Part model, mm, in its own coordinate system. A direction names the side the tool comes from. Give positions to 0.01 mm unless a question says otherwise; leave off trailing zeros. Write each loop counter-clockwise with the first axis right and the second up, starting at its lowest first coordinate (ties: lowest second). Pieces come first, ordered by that corner, then holes. Notation, with made-up numbers: (88.25, 33.5) - (105.25, 33.5) arc R27 cw to (105.25, 59.5) - close; hole circle Ø2 at (-11, 34.5). An arc over 180 degrees is marked (long way). Answer in a Markdown table with one row per item. Add a question column.
1. Band-saw the part on A-A on y = 45. Write the cut outline in (x, z), plus the area to 3 significant figures.
2. Band-saw the part on B-B on y = -60.18. Write the cut outline in (x, z).
3. Which spindle directions (+Z, -Z, +X, -X, +Y, -Y) get a long thin tool onto all of the face, cutting with end or side? Do faces 1 (the flat face through (-16, 17, -11)), 2 (the cylindrical face through (-16.507, 73.676, -13.218)), 3 (the cylindrical face through (-10.5, 64.9, -0.5)), 4 (the flat face through (16.49, 3.77, -7.83)). Say none if no direction does.
4. Band-saw the part on C-C on x = 3.5. Write the cut outline in (y, z), plus the area to 3 significant figures.
5. Drop flat-ended pins along their axis: pin 1 Ø12 at (x, y) = (-11, -49.5) entering from +Z; pin 2 Ø1.1 at (y, z) = (-62, -0.5) entering from -X; pin 3 Ø0.8 at (x, y) = (-16.5, 18) entering from +Z; pin 4 Ø1 at (x, z) = (16, -2.5) entering from -Y. Give the stop position or say it passes through.
6. Probe line 1 along X through (y, z) = (-70.18, -0.8); line 2 along X through (y, z) = (60, -7.75); line 3 along Z through (x, y) = (-12, -53.5). List the from-to ranges inside material, lowest first.
7. Pull direction Z, two halves, no side cores. Call faces 5 (the flat face through (-16.51, 3.77, -7.83)), 6 (the cylindrical face through (10.5, 25.1, -0.5)), 7 (the flat face through (14, 1, -1)): released by +Z, released by -Z, zero draft, split by the parting line, or undercut.
8. Band-saw the part on D-D on z = -12.75. Write the cut outline in (x, y), plus the area to 3 significant figures.
```python
from build123d import *

# Parameters (mm, degrees)
SKETCH1_R                  = 6.5
BASE_FLANGE1_DEPTH         = 1
FILLET1_R                  = 5
SKETCHED_START             = 16.78876
SKETCHED_BEND1_OUTLINE_W   = 115.36
SKETCHED_BEND1_OUTLINE_H   = 1
SKETCHED_BEND1_DEPTH       = 13.21124
SKETCHED_START_2           = -30
SKETCHED_BEND1_2_OUTLINE_W = 115.36
SKETCHED_BEND1_2_OUTLINE_H = 1
SKETCHED_BEND1_2_DEPTH     = 13.18876
SKETCHED_START_3           = 16
SKETCHED_BEND1_3_DEPTH     = 0.0274
SKETCHED_START_4           = -16.01124
SKETCHED_BEND1_4_DEPTH     = 0.01124
SKETCHED_START_5           = -17
SKETCHED_BEND1_5_DEPTH     = 2
SKETCHED_START_6           = 15
SKETCHED_BEND1_6_DEPTH     = 2
SKETCHED_START_7           = -40.18
SKETCHED_BEND1_7_DEPTH     = 115.36
F_4_CLEARANCE_HOLE1_D      = 3.2639
FILLET2_R                  = 1
F_6_CLEARANCE_HOLE2_D      = 3.7973
CUT_EXTRUDE1_DEPTH         = 10


with BuildPart() as part:
    # Base-Flange1: sheet metal written as solids
    # Sketch1 → Base-Flange1 (new body)
    with BuildSketch(Plane.XY):
        Polygon((-30, 75.18), (30, 75.18), (30, -40.18), (15, -40.18), (15, -75.18), (-15, -75.18), (-15, -40.18), (-30, -40.18), align=None)
        with Locations((0, -60.18)):
            Circle(SKETCH1_R, mode=Mode.SUBTRACT)
        Polygon((-26, 60.18), (-19, 54.18), (-19, 36.18), (-26, 30.18), align=None, mode=Mode.SUBTRACT)
        Polygon((-26, 24.18), (-19, 30.18), (-19, 0.18), (-26, 6.18), align=None, mode=Mode.SUBTRACT)
        Polygon((-26, -29.82), (-26, 0.18), (-19, -5.82), (-19, -23.82), align=None, mode=Mode.SUBTRACT)
        Polygon((19, -23.82), (26, -29.82), (26, 0.18), (19, -5.82), align=None, mode=Mode.SUBTRACT)
        Polygon((19, 0.18), (26, 6.18), (26, 24.18), (19, 30.18), align=None, mode=Mode.SUBTRACT)
        Polygon((19, 36.18), (26, 30.18), (26, 60.18), (19, 54.18), align=None, mode=Mode.SUBTRACT)
    extrude(amount=-BASE_FLANGE1_DEPTH)

    # Fillet1
    fillet1_edges = [part.edges().sort_by_distance(p)[0] for p in [
        (-30, 75.18, -0.5),
        (30, 75.18, -0.5),
        (30, -40.18, -0.5),
        (15, -75.18, -0.5),
        (-15, -75.18, -0.5),
        (-30, -40.18, -0.5),
    ]]
    fillet(fillet1_edges, radius=FILLET1_R)

    # Sketched Bend1: read off the stored shape, not the designer's step
    # Sketched Bend1 outline → Sketched Bend1 (cut)
    with BuildSketch(Plane.YZ.offset(SKETCHED_START)):
        with Locations((17.5, -0.5)):
            Rectangle(SKETCHED_BEND1_OUTLINE_W, SKETCHED_BEND1_OUTLINE_H)
    extrude(amount=SKETCHED_BEND1_DEPTH, mode=Mode.SUBTRACT)

    # Sketched Bend1 2 outline → Sketched Bend1 2 (cut)
    with BuildSketch(Plane.YZ.offset(SKETCHED_START_2)):
        with Locations((17.5, -0.5)):
            Rectangle(SKETCHED_BEND1_2_OUTLINE_W, SKETCHED_BEND1_2_OUTLINE_H)
    extrude(amount=SKETCHED_BEND1_2_DEPTH, mode=Mode.SUBTRACT)

    # Sketched Bend1 3 outline → Sketched Bend1 3 (add)
    with BuildSketch(Plane.YZ.offset(SKETCHED_START_3)):
        with BuildLine():
            Line((75.18, -9.64380551), (75.18, -1))
            Line((75.18, -1), (-40.18, -1))
            Line((-40.18, -1), (-40.18, -9.64380551))
            ThreePointArc((-40.18, -9.64380551), (-38.715533906, -13.179339416), (-35.18, -14.64380551))
            Line((-35.18, -14.64380551), (70.18, -14.64380551))
            ThreePointArc((70.18, -14.64380551), (73.715533906, -13.179339416), (75.18, -9.64380551))
        make_face()
        Polygon((-23.82, -3.64380551), (-5.82, -3.64380551), (0.18, -10.64380551), (-29.82, -10.64380551), align=None, mode=Mode.SUBTRACT)
        Polygon((0.18, -3.64380551), (30.18, -3.64380551), (24.18, -10.64380551), (6.18, -10.64380551), align=None, mode=Mode.SUBTRACT)
        Polygon((36.18, -3.64380551), (54.18, -3.64380551), (60.18, -10.64380551), (30.18, -10.64380551), align=None, mode=Mode.SUBTRACT)
    extrude(amount=SKETCHED_BEND1_3_DEPTH)

    # Sketched Bend1 4 outline → Sketched Bend1 4 (add)
    with BuildSketch(Plane.YZ.offset(SKETCHED_START_4)):
        with BuildLine():
            Line((75.18, -9.64380551), (75.18, -1))
            Line((75.18, -1), (-40.18, -1))
            Line((-40.18, -1), (-40.18, -9.64380551))
            ThreePointArc((-40.18, -9.64380551), (-38.715533906, -13.179339416), (-35.18, -14.64380551))
            Line((-35.18, -14.64380551), (70.18, -14.64380551))
            ThreePointArc((70.18, -14.64380551), (73.715533906, -13.179339416), (75.18, -9.64380551))
        make_face()
        Polygon((-23.82, -3.64380551), (-5.82, -3.64380551), (0.18, -10.64380551), (-29.82, -10.64380551), align=None, mode=Mode.SUBTRACT)
        Polygon((0.18, -3.64380551), (30.18, -3.64380551), (24.18, -10.64380551), (6.18, -10.64380551), align=None, mode=Mode.SUBTRACT)
        Polygon((36.18, -3.64380551), (54.18, -3.64380551), (60.18, -10.64380551), (30.18, -10.64380551), align=None, mode=Mode.SUBTRACT)
    extrude(amount=SKETCHED_BEND1_4_DEPTH)

    # Sketched Bend1 5 outline → Sketched Bend1 5 (add)
    with BuildSketch(Plane.YZ.offset(SKETCHED_START_5)):
        with BuildLine():
            Line((75.18, -9.64380551), (75.18, -1))
            Line((75.18, -1), (-40.18, -1))
            Line((-40.18, -1), (-40.18, -9.64380551))
            ThreePointArc((-40.18, -9.64380551), (-38.715533906, -13.179339416), (-35.18, -14.64380551))
            Line((-35.18, -14.64380551), (70.18, -14.64380551))
            ThreePointArc((70.18, -14.64380551), (73.715533906, -13.179339416), (75.18, -9.64380551))
        make_face()
        Polygon((-23.82, -3.64380551), (-5.82, -3.64380551), (0.18, -10.64380551), (-29.82, -10.64380551), align=None, mode=Mode.SUBTRACT)
        Polygon((0.18, -3.64380551), (30.18, -3.64380551), (24.18, -10.64380551), (6.18, -10.64380551), align=None, mode=Mode.SUBTRACT)
        Polygon((36.18, -3.64380551), (54.18, -3.64380551), (60.18, -10.64380551), (30.18, -10.64380551), align=None, mode=Mode.SUBTRACT)
    extrude(amount=SKETCHED_BEND1_5_DEPTH)

    # Sketched Bend1 6 outline → Sketched Bend1 6 (add)
    with BuildSketch(Plane.YZ.offset(SKETCHED_START_6)):
        with BuildLine():
            Line((75.18, -9.64380551), (75.18, -1))
            Line((75.18, -1), (-40.18, -1))
            Line((-40.18, -1), (-40.18, -9.64380551))
            ThreePointArc((-40.18, -9.64380551), (-38.715533906, -13.179339416), (-35.18, -14.64380551))
            Line((-35.18, -14.64380551), (70.18, -14.64380551))
            ThreePointArc((70.18, -14.64380551), (73.715533906, -13.179339416), (75.18, -9.64380551))
        make_face()
        Polygon((-23.82, -3.64380551), (-5.82, -3.64380551), (0.18, -10.64380551), (-29.82, -10.64380551), align=None, mode=Mode.SUBTRACT)
        Polygon((0.18, -3.64380551), (30.18, -3.64380551), (24.18, -10.64380551), (6.18, -10.64380551), align=None, mode=Mode.SUBTRACT)
        Polygon((36.18, -3.64380551), (54.18, -3.64380551), (60.18, -10.64380551), (30.18, -10.64380551), align=None, mode=Mode.SUBTRACT)
    extrude(amount=SKETCHED_BEND1_6_DEPTH)

    # Sketched Bend1 7 outline → Sketched Bend1 7 (cut)
    with BuildSketch(Plane(origin=(0, 0, 0), x_dir=(1, 0, 0), z_dir=(0, 1, 0)).offset(SKETCHED_START_7)):
        with BuildLine():
            ThreePointArc((-16, 2), (-15.707106781, 1.292893219), (-15, 1))
            Line((-15, 1), (-15, 14.64380551))
            Line((-15, 14.64380551), (-16, 14.64380551))
            Line((-16, 14.64380551), (-16, 2))
        make_face()
        with BuildLine():
            ThreePointArc((17, 2), (16.414213562, 0.585786438), (15, 0))
            Line((15, 0), (16.78876, 0))
            Line((16.78876, 0), (16.78876, 1))
            Line((16.78876, 1), (17, 1))
            Line((17, 1), (17, 2))
        make_face()
        with BuildLine():
            ThreePointArc((-15, 0), (-16.414213562, 0.585786438), (-17, 2))
            Line((-17, 2), (-17, 1))
            Line((-17, 1), (-16.81124, 1))
            Line((-16.81124, 1), (-16.81124, 0))
            Line((-16.81124, 0), (-15, 0))
        make_face()
        with BuildLine():
            ThreePointArc((15, 1), (15.707106781, 1.292893219), (16, 2))
            Line((16, 2), (16, 14.64380551))
            Line((16, 14.64380551), (15, 14.64380551))
            Line((15, 14.64380551), (15, 1))
        make_face()
    extrude(amount=SKETCHED_BEND1_7_DEPTH, mode=Mode.SUBTRACT)

    # #4 Clearance Hole1 (through all)
    with Locations(Plane.XY):
        with Locations((0, -50.18), (0, -70.18)):
            Hole(F_4_CLEARANCE_HOLE1_D / 2)

    # Fillet2
    fillet2_edges = [part.edges().sort_by_distance(p)[0] for p in [
        (-16.5, 36.18, -3.64380551),
        (-16.5, 30.18, -10.64380551),
        (-16.5, 60.18, -10.64380551),
        (-16.5, 54.18, -3.64380551),
        (-16.5, 30.18, -3.64380551),
        (-16.5, 0.18, -3.64380551),
        (-16.5, 6.18, -10.64380551),
        (-16.5, 24.18, -10.64380551),
        (-16.5, -29.82, -10.64380551),
        (-16.5, 0.18, -10.64380551),
        (-16.5, -5.82, -3.64380551),
        (-16.5, -23.82, -3.64380551),
        (16.5, -29.82, -10.64380551),
        (16.5, -23.82, -3.64380551),
        (16.5, -5.82, -3.64380551),
        (16.5, 0.18, -10.64380551),
        (16.5, 6.18, -10.64380551),
        (16.5, 0.18, -3.64380551),
        (16.5, 30.18, -3.64380551),
        (16.5, 24.18, -10.64380551),
        (16.5, 30.18, -10.64380551),
        (16.5, 36.18, -3.64380551),
        (16.5, 54.18, -3.64380551),
        (16.5, 60.18, -10.64380551),
    ]]
    fillet(fillet2_edges, radius=FILLET2_R)

    # #6 Clearance Hole2 (through all)
    with Locations(Plane.XY):
        with Locations((-8, 12), (8, 12), (0, -10.5), (-8, -33), (8, -33)):
            Hole(F_6_CLEARANCE_HOLE2_D / 2)

    # Sketch13 → Cut-Extrude1 (cut)
    with BuildSketch(Plane.XY):
        with BuildLine():
            Line((-7.5, 3), (7.5, 3))
            ThreePointArc((7.5, 3), (10.5, 0), (7.5, -3))
            Line((7.5, -3), (-7.5, -3))
            ThreePointArc((-7.5, -3), (-10.5, 0), (-7.5, 3))
        make_face()
        with BuildLine():
            Line((-7.5, -17), (7.5, -17))
            ThreePointArc((7.5, -17), (10.5, -20), (7.5, -23))
            Line((7.5, -23), (-7.5, -23))
            ThreePointArc((-7.5, -23), (-10.5, -20), (-7.5, -17))
        make_face()
        with BuildLine():
            Line((-7.5, 28), (7.5, 28))
            ThreePointArc((7.5, 28), (10.5, 25), (7.5, 22))
            Line((7.5, 22), (-7.5, 22))
            ThreePointArc((-7.5, 22), (-10.5, 25), (-7.5, 28))
        make_face()
        with BuildLine():
            Line((-7.5, 48), (7.5, 48))
            ThreePointArc((7.5, 48), (10.5, 45), (7.5, 42))
            Line((7.5, 42), (-7.5, 42))
            ThreePointArc((-7.5, 42), (-10.5, 45), (-7.5, 48))
        make_face()
        with BuildLine():
            Line((-7.5, 68), (7.5, 68))
            ThreePointArc((7.5, 68), (10.5, 65), (7.5, 62))
            Line((7.5, 62), (-7.5, 62))
            ThreePointArc((-7.5, 62), (-10.5, 65), (-7.5, 68))
        make_face()
    extrude(amount=-CUT_EXTRUDE1_DEPTH, mode=Mode.SUBTRACT)


solid = part.part
```
Values:
| question | item | result |
|---|---|---|
| 1 | outline | (-17, -14.64) - (-16, -14.64) - (-16, -10.64) - (-17, -10.64) - close; (-17, -3.64) - (-16, -3.64) - (-16, -2) arc R1 cw to (-15, -1) - (-10.5, -1) - (-10.5, 0) - (-15, 0) arc R2 ccw to (-17, -2) - close; (10.5, -1) - (15, -1) arc R1 cw to (16, -2) - (16, -3.64) - (17, -3.64) - (17, -2) arc R2 ccw to (15, 0) - (10.5, 0) - close; (16, -14.64) - (17, -14.64) - (17, -10.64) - (16, -10.64) - close |
| 1 | area | 25.0 mm² |
| 2 | outline | (-15, -1) - (-6.5, -1) - (-6.5, 0) - (-15, 0) - close; (6.5, -1) - (15, -1) - (15, 0) - (6.5, 0) - close |
| 3 | face 1 | -Z, +Y, -Y |
| 3 | face 2 | -Z, +X, -X, +Y |
| 3 | face 3 | +Z, -Z |
| 3 | face 4 | +X, -X |
| 4 | outline | (-75.18, -1) - (-65.66, -1) - (-65.66, 0) - (-75.18, 0) - close; (-54.7, -1) - (-23, -1) - (-23, 0) - (-54.7, 0) - close; (-17, -1) - (-3, -1) - (-3, 0) - (-17, 0) - close; (3, -1) - (22, -1) - (22, 0) - (3, 0) - close; (28, -1) - (42, -1) - (42, 0) - (28, 0) - close; (48, -1) - (62, -1) - (62, 0) - (48, 0) - close; (68, -1) - (75.18, -1) - (75.18, 0) - (68, 0) - close |
| 4 | area | 109 mm² |
| 5 | pin 1 | stops at z = 0 |
| 5 | pin 2 | stops at x = -15 |
| 5 | pin 3 | stops at z = -0.33 |
| 5 | pin 4 | stops at y = -40.18 |
| 6 | line 1 | x = -15 to -1.63, 1.63 to 15 |
| 6 | line 2 | x = -17 to -16, 16 to 17 |
| 6 | line 3 | z = -1 to 0 |
| 7 | face 5 | undercut |
| 7 | face 6 | zero draft |
| 7 | face 7 | released by -Z |
| 8 | outline | (-17, -39.1) - (-16, -39.1) - (-16, 74.1) - (-17, 74.1) - close; (16, -39.1) - (17, -39.1) - (17, 74.1) - (16, 74.1) - close |
| 8 | area | 226 mm² |
